The listing builds one solid part. Answer for the finished solid, in the listing's coordinates (mm). A direction names the side the tool comes from. Round coordinates to 2 decimals unless told otherwise and drop trailing zeros. Loops run counter-clockwise (first coordinate to the right, second up) from the corner with the lowest first, then second, coordinate; pieces in that order, holes last. Notation, with made-up numbers: (23.25, 41) -> (68.25, 41) arc R18 ccw to (68.25, 75) -> close; hole circle Ø1 at (37.25, -32). An arc over 180 degrees is marked (long way). Answer in a Markdown table with one row per item. Add a question column.
```python
from build123d import *

# Parameters (mm, degrees)
SKETCH1_R           = 25.65
SKETCH1_R_2         = 1.45
BOSS_EXTRUDE1_DEPTH = 10
CUT_EXTRUDE1_DEPTH  = 7.5


with BuildPart() as part:
    # Sketch1 → Boss-Extrude1 (new body)
    with BuildSketch(Plane.XY):
        Circle(SKETCH1_R)
        with Locations((0, -22.65)):
            Circle(SKETCH1_R_2, mode=Mode.SUBTRACT)
        with Locations((22.65, 0)):
            Circle(SKETCH1_R_2, mode=Mode.SUBTRACT)
        with Locations((0, 22.65)):
            Circle(SKETCH1_R_2, mode=Mode.SUBTRACT)
        with Locations((-22.65, 0)):
            Circle(SKETCH1_R_2, mode=Mode.SUBTRACT)
    extrude(amount=BOSS_EXTRUDE1_DEPTH)

    # Sketch2 → Cut-Extrude1 (cut)
    with BuildSketch(Plane.XY.offset(10)):
        Polygon((1.682914139, 15.047232304), (15.047232304, 1.682914139), (17.380684682, 4.016366517), (11.264211024, 10.132840174), (12.890556621, 11.759185771), (11.759185771, 12.890556621), (10.132840174, 11.264211024), (4.016366517, 17.380684682), align=None)
    extrude(amount=-CUT_EXTRUDE1_DEPTH, mode=Mode.SUBTRACT)


solid = part.part
```
Item 1: The mould has two halves that part along X. Classify faces 3 (the cylindrical face through (-3.34, 25.43, 4.93)), 4 (the flat face through (0, 0, 10)), 5 (the flat face through (2.866, 16.23, 6.302)), 6 (the flat face through (9, 10, 2.5)): +X half, -X half, draft (parallel to the pull), parting line (faces both ways), or undercut.
Item 2: Section B-B, the plane z = 7.25 is taken. Write down the section's boundary in (x, y), and give its area (3 significant figures).
Item 3: Section D-D, the plane x = -22.65 is taken. Write down the section's boundary in (y, z).
Item 4: Consider L1, parallel to Y at x = 0, z = 6.25; L2, parallel to X at y = 0.5, z = 5; L3, parallel to X at y = 9, z = 2.75. Determine where each line is inside the solid, lowest interval first. Write a range as from..to.
Item 5: For faces 1 (the flat face through (8.27, 8.46, 6.3)), 2 (the cylindrical face through (-24.1, 0.06, 4.93)), determine the directions among +Z, -Z, +X, -X, +Y, -Y from which every point of the face is accessible in a straight line to the end or side of a thin tool.
Item 6: Section C-C, the plane z = 1.5 is taken. Write down the section's boundary in (x, y).
Item 7: Flat-ended cylindrical pins translate along their axes: P1, Ø1, axis at x = 20, z = 6, coming from the -Y side; P2, Ø6, axis at y = 13.5, z = 9, coming from the -X side; P3, Ø5, axis at y = -11, z = 8.5, coming from the +X side. Find the tip coordinate at first contact, or state that the pin passes through.
Item 8: Section A-A, the plane y = 0 is taken. Write down the section's boundary in (x, z).
Here are the results:
| question | item | result |
|---|---|---|
| 1 | face 3 | parting line |
| 1 | face 4 | draft |
| 1 | face 5 | undercut |
| 1 | face 6 | undercut |
| 2 | outline | circle Ø51.3 at (0, 0); hole circle Ø2.9 at (-22.65, 0); hole circle Ø2.9 at (0, -22.65); hole circle Ø2.9 at (0, 22.65); hole (1.68, 15.05) -> (15.05, 1.68) -> (17.38, 4.02) -> (11.26, 10.13) -> (12.89, 11.76) -> (11.76, 12.89) -> (10.13, 11.26) -> (4.02, 17.38) -> close; hole circle Ø2.9 at (22.65, 0) |
| 2 | area | 1,970 mm² |
| 3 | outline | (-12.04, 0) -> (-1.45, 0) -> (-1.45, 10) -> (-12.04, 10) -> close; (1.45, 0) -> (12.04, 0) -> (12.04, 10) -> (1.45, 10) -> close |
| 4 | L1 | y = -25.65..-24.1, -21.2..21.2, 24.1..25.65 |
| 4 | L2 | x = -25.65..-24.01, -21.29..21.29, 24.01..25.65 |
| 4 | L3 | x = -24.02..7.73, 12.4..24.02 |
| 5 | face 1 | +Z |
| 5 | face 2 | +Z, -Z |
| 6 | outline | circle Ø51.3 at (0, 0); hole circle Ø2.9 at (-22.65, 0); hole circle Ø2.9 at (0, -22.65); hole circle Ø2.9 at (0, 22.65); hole circle Ø2.9 at (22.65, 0) |
| 7 | P1 | stops at y = -16.66 |
| 7 | P2 | stops at x = -23.4 |
| 7 | P3 | stops at x = 24.2 |
| 8 | outline | (-25.65, 0) -> (-24.1, 0) -> (-24.1, 10) -> (-25.65, 10) -> close; (-21.2, 0) -> (21.2, 0) -> (21.2, 10) -> (-21.2, 10) -> close; (24.1, 0) -> (25.65, 0) -> (25.65, 10) -> (24.1, 10) -> close |
